```python
from build123d import *

# Parameters (mm, degrees)
BOSS_EXTRUDE2_DEPTH = 8
SKETCH2_R           = 1.5
CUT_EXTRUDE1_DEPTH  = 20


with BuildPart() as part:
    # Sketch1 → Boss-Extrude2 (new body)
    with BuildSketch(Plane(origin=(0, 0, 0), x_dir=(1, 0, 0), z_dir=(0, 1, 0))):
        Polygon((0, 0), (33, 0), (33, 21.667134547), (0, 35), align=None)
    extrude(amount=BOSS_EXTRUDE2_DEPTH)

    # Sketch2 → Cut-Extrude1 (cut)
    with BuildSketch(Plane(origin=(0, 0, 0), x_dir=(0, 0, -1), z_dir=(1, 0, 0))):
        with Locations((17.5, 4)):
            Circle(SKETCH2_R)
    extrude(amount=CUT_EXTRUDE1_DEPTH, mode=Mode.SUBTRACT)


solid = part.part
```
The listing builds one solid part. Answer for the finished solid, in the listing's coordinates (mm). A direction names the side the tool comes from. Round coordinates to 2 decimals unless told otherwise and drop trailing zeros. Write each loop counter-clockwise with the first axis right and the second up, starting at its lowest first coordinate (ties: lowest second). Pieces come first, ordered by that corner, then holes. Notation, with made-up numbers: (-1, -0.5) -> (17, -0.5) arc R24 cw to (17, 10.5) -> close; hole circle Ø7 at (-7.75, 83). An arc over 180 degrees is marked (long way). Answer as a JSON object with one key per item and string values. Group by question number.
Q1. Section A-A (y = 4) is taken. Write down the section's boundary in (x, z).
Q2. Section B-B (z = -17.5) is taken. Write down the section's boundary in (x, y), plus the area to 3 significant figures.
Q3. Straight lines are drawn through the part: line 1 along Y through (x, z) = (14.5, -17.5); line 2 along Y through (x, z) = (5, -17); line 3 along Z through (x, y) = (3, 4.5). For each, find the intervals that lie inside material, in ascending order.
Q4. Section C-C (x = 5.5) is taken. Write down the section's boundary in (y, z), plus the area to 3 significant figures.
Q5. Section D-D (x = 17.5) is taken. Write down the section's boundary in (y, z).
Q6. Determine the mould class of faces 3 (the face through (16, 0, -14)), 4 (the face through (16, 8, -14)), 5 (the face through (20, 4, -17)) for opening direction Y: pulls with the +Y half, pulls with the -Y half, needs draft (parallel to the pull), parting line crosses it, or undercut.
Q7. Each of these flat-tipped pins is pushed along its axis until it touches: pin 1 Ø1.5 at (y, z) = (4.5, -17) entering from -X; pin 2 Ø1 at (y, z) = (4.5, -26.5) entering from +X; pin 3 Ø1 at (y, z) = (4, -24.5) entering from +X; pin 4 Ø3 at (x, z) = (25.5, -27.5) entering from -Y. Where does it stop, or does it pass through?
Q8. Which of the six approach directions +Z, -Z, +X, -X, +Y, -Y give full straight-line access (tool end or side, diameter ignored) to faces 1 (the face through (10, 4, -16)), 2 (the face through (16, 4, 0))?
Check values:
{
 "1": {"outline": "(0, -35) -> (33, -21.67) -> (33, 0) -> (0, 0) -> (0, -16) -> (20, -16) -> (20, -19) -> (0, -19) -> close"},
 "2": {"outline": "(0, 0) -> (33, 0) -> (33, 8) -> (0, 8) -> (0, 5.5) -> (20, 5.5) -> (20, 2.5) -> (0, 2.5) -> close", "area": "204 mm^2"},
 "3": {"line 1": "0 to 2.5, 5.5 to 8", "line 2": "0 to 2.59, 5.41 to 8", "line 3": "-33.79 to -18.91, -16.09 to 0"},
 "4": {"outline": "(0, -32.78) -> (8, -32.78) -> (8, 0) -> (0, 0) -> close; hole circle Ø3 at (4, -17.5)", "area": "255 mm^2"},
 "5": {"outline": "(0, -27.93) -> (8, -27.93) -> (8, 0) -> (0, 0) -> close; hole circle Ø3 at (4, -17.5)"},
 "6": {"face 3": "pulls with the -Y half", "face 4": "pulls with the +Y half", "face 5": "undercut"},
 "7": {"pin 1": "x = 20", "pin 2": "x = 22.28", "pin 3": "x = 27.23", "pin 4": "through"},
 "8": {"face 1": "-X", "face 2": "+Z, +X, -X, +Y, -Y"}
}
